Can you work these out from the model? Positions are in its coordinate system, mm. A direction names the side the tool comes from. Give positions to 0.01 mm unless a question says otherwise; leave off trailing zeros. Order: outer loops, then holes, each group sorted by start corner. A loop starts at its lowest first (then second) coordinate and runs counter-clockwise, first axis right, second up. Notation, with made-up numbers: M 13.25,-29.75 L 39.25,-29.75 A23 cw 39.25,3.25 Z; hole C 34.25,-9.5 d6. An arc over 180 degrees is marked long. One line per question, with ' | ' between items. Start each with the question number.
1) Please list where these lines run through material, in increasing order: line 1 along Y through (x, z) = (4, -2); line 2 along Y through (x, z) = (8, 8); line 3 along Y through (x, z) = (3.5, 7.75). Write a range as [from, to].
2) If we section it at C-C, the plane x = 6: State how many separate pieces and enclosed holes the cut face has, plus the area to 3 significant figures.
3) For faces 1 (the flat face through (3.5, 2, -1)), 2 (the flat face through (6, 3.85, -1)), 3 (the flat face through (1.08, 12, 14)), 4 (the flat face through (6, -0.25, -1)), 5 (the flat face through (8.5, 2, -1)), which set-ups out of +Z, -Z, +X, -X, +Y, -Y let a thin tool reach every point of the face, with its end or its side?
4) If we section it at D-D, the plane x = 2.25: Please give me the cut outline in (y, z), plus the area to 3 significant figures.
5) I'm going to push flat-ended pins straight in: pin 1 Ø3 at (y, z) = (1.5, 7) entering from +X; pin 2 Ø0.7 at (y, z) = (8.5, -4.5) entering from +X; pin 3 Ø0.7 at (y, z) = (1.5, -6.5) entering from -X. Where does each tip first touch, or does it pass through?
6) If we section it at B-B, the plane z = 1: Please give me the cut outline in (x, y), plus the area to 3 significant figures.
7) If we section it at A-A, the plane z = -5.4: Please give me the cut outline in (x, y), plus the area to 3 significant figures.
8) Thinking about a two-plate mould opening in Z: for faces 6 (the cylindrical face through (5.9, 15.4, 15.3)), 7 (the flat face through (7, -0.8, 2)), 8 (the cylindrical face through (5.263, 8.596, -4.724)), 9 (the flat face through (6, 17.2, 7)), which applies, +Z half, -Z half, draft (parallel to the pull), parting line (faces both ways), or undercut?
```python
from build123d import *

# Parameters (mm, degrees)
SKETCH001_W      = 9
SKETCH001_H      = 3
EXTRUDE001_DEPTH = 0.8
SKETCH002_W      = 9
SKETCH002_H      = 3
EXTRUDE002_DEPTH = 0.8
EXTRUDE005_DEPTH = 15.15
EXTRUDE004_DEPTH = 21.28
SKETCH003_W      = 15.15
SKETCH003_H      = 21.28
EXTRUDE003_DEPTH = 2.15
EXTRUDE006_DEPTH = 6
EXTRUDE007_DEPTH = 9.84
SKETCH008_W      = 5
SKETCH008_H      = 4.1
EXTRUDE008_DEPTH = 1.8
SKETCH010_R      = 1
EXTRUDE010_DEPTH = 8
SKETCH009_W      = 4.8
SKETCH009_H      = 0.64
EXTRUDE009_DEPTH = 7.2
SKETCH_W         = 12
SKETCH_H         = 17.2
EXTRUDE_DEPTH    = 11


with BuildPart() as extrude001:
    # Sketch001 (on Face1 of Extrude) → Extrude001 (new body)
    with BuildSketch(Plane.XZ):
        with Locations((7.5, 1.5)):
            Rectangle(SKETCH001_W, SKETCH001_H)
    extrude(amount=EXTRUDE001_DEPTH)


with BuildPart() as extrude002:
    # Sketch002 (on Face3 of Extrude) → Extrude002 (new body)
    with BuildSketch(Plane(origin=(0, 17.2, 0), x_dir=(-1, 0, 0), z_dir=(0, 1, 0))):
        with Locations((-7.5, 1.5)):
            Rectangle(SKETCH002_W, SKETCH002_H)
    extrude(amount=EXTRUDE002_DEPTH)


with BuildPart() as extrude005:
    # Sketch005 (on Face3 of Extrude003) → Extrude005 (new body)
    with BuildSketch(Plane.YZ.offset(13.575)):
        Polygon((19.24, 13.15), (17.74, 13.15), (19.24, 12.5), align=None)
        Polygon((-2.04, 13.15), (-0.54, 13.15), (-2.04, 12.5), align=None)
    extrude(amount=-EXTRUDE005_DEPTH)


with BuildPart() as fusion:
    # Sketch004 (on Face4 of Extrude003) → Extrude004 (new body)
    with BuildSketch(Plane(origin=(0, 19.24, 0), x_dir=(-1, 0, 0), z_dir=(0, 1, 0))):
        Polygon((-12.075, 13.15), (-13.575, 12.5), (-13.575, 13.15), align=None)
        Polygon((1.575, 13.15), (1.575, 12.5), (0.075, 13.15), align=None)
    extrude(amount=-EXTRUDE004_DEPTH)

    # Fusion: union Extrude005
    add(extrude005.part)


with BuildPart() as cut:
    # Sketch003 (on Face6 of Extrude) → Extrude003 (new body)
    with BuildSketch(Plane.XY.offset(11)):
        with Locations((6, 8.6)):
            Rectangle(SKETCH003_W, SKETCH003_H)
    extrude(amount=EXTRUDE003_DEPTH)

    # Cut: cut Fusion
    add(fusion.part, mode=Mode.SUBTRACT)


with BuildPart() as extrude006:
    # Sketch006 (on Face2 of Extrude) → Extrude006 (new body)
    with BuildSketch(Plane.YZ.offset(3)):
        Polygon((17.2, 3), (18.2, 7.6), (17.2, 11), (18, 11), (19, 7.6), (18, 3), align=None)
        Polygon((-0.8, 3), (-1.8, 7.6), (-0.8, 11), (0, 11), (-1, 7.6), (0, 3), align=None)
    extrude(amount=EXTRUDE006_DEPTH)


with BuildPart() as extrude007:
    # Sketch007 (on Face4 of Extrude) → Extrude007 (new body)
    with BuildSketch(Plane(origin=(1.08, 0, 0), x_dir=(0, -1, 0), z_dir=(-1, 0, 0))):
        with BuildLine():
            Line((-0.7, 11), (-0.7, 13.3))
            ThreePointArc((-13.9, 17.04), (-7.559803, 14.253048), (-0.7, 13.3))
            ThreePointArc((-13.9, 17.04), (-15.395706, 15.306052), (-16.5, 13.3))
            Line((-16.5, 11), (-16.5, 13.3))
            Line((-16.5, 11), (-0.7, 11))
        make_face()
    extrude(amount=-EXTRUDE007_DEPTH)


with BuildPart() as extrude008:
    # Sketch008 (on Face5 of Extrude) → Extrude008 (new body)
    with BuildSketch(Plane(origin=(0, 0, 0), x_dir=(1, 0, 0), z_dir=(0, 0, -1))):
        with Locations((6, -1.8)):
            Rectangle(SKETCH008_W, SKETCH008_H)
        with Locations((6, -8.6)):
            Rectangle(SKETCH008_W, SKETCH008_H)
        with Locations((6, -15.4)):
            Rectangle(SKETCH008_W, SKETCH008_H)
    extrude(amount=EXTRUDE008_DEPTH)


with BuildPart() as extrude010:
    # Sketch010 (on Face10 of Extrude009) → Extrude010 (new body)
    with BuildSketch(Plane.XZ.offset(-1.48)):
        with Locations((6, -5.4)):
            Circle(SKETCH010_R)
        Polygon((3.6, -9), (4.2, -9), (3.6, -8.4), align=None)
        Polygon((8.4, -9), (7.8, -9), (8.4, -8.4), align=None)
    extrude(amount=-EXTRUDE010_DEPTH)


with BuildPart() as cut001:
    # Sketch009 (on Face6 of Extrude008) → Extrude009 (new body)
    with BuildSketch(Plane(origin=(0, 0, -1.8), x_dir=(1, 0, 0), z_dir=(0, 0, -1))):
        with Locations((6, -1.8)):
            Rectangle(SKETCH009_W, SKETCH009_H)
        with Locations((6, -8.6)):
            Rectangle(SKETCH009_W, SKETCH009_H)
    extrude(amount=EXTRUDE009_DEPTH)

    # Cut001: cut Extrude010
    add(extrude010.part, mode=Mode.SUBTRACT)


with BuildPart() as fusion001:
    # Sketch → Extrude (new body)
    with BuildSketch(Plane.XY):
        with Locations((6, 8.6)):
            Rectangle(SKETCH_W, SKETCH_H)
    extrude(amount=EXTRUDE_DEPTH)

    # Fusion001: union Extrude001, Extrude002, Cut, Extrude006, Extrude007, Extrude008, Cut001
    add(extrude001.part)
    add(extrude002.part)
    add(cut.part)
    add(extrude006.part)
    add(extrude007.part)
    add(extrude008.part)
    add(cut001.part)


solid = fusion001.part
```
Results found:
1) line 1: y = [1.48, 2.12], [8.28, 8.92] | line 2: y = [-1.68, -0.88], [0, 17.2], [18.08, 18.88] | line 3: y = [-1.76, -0.96], [0, 17.2], [18.16, 18.96]
2) separate pieces: 3 | enclosed holes: 2 | area: 304 mm²
3) face 1: -Z, -X, +Y, -Y | face 2: -Z, +X, -X | face 3: +Z, -X, +Y, -Y | face 4: -Z, +X, -X, -Y | face 5: -Z, +X, +Y, -Y
4) outline: M -2.04,11 L 0,11 L 0,0 L 17.2,0 L 17.2,11 L 19.24,11 L 19.24,12.5 L 17.74,13.15 L 16.5,13.15 L 16.5,13.3 A11 ccw 13.9,17.04 A25.16 cw 0.7,13.3 L 0.7,13.15 L -0.54,13.15 L -2.04,12.5 Z | area: 258 mm²
5) pin 1: stops at x = 12 | pin 2: stops at x = 8.4 | pin 3: stops at x = 3.6
6) outline: M 0,0 L 3,0 L 3,-0.8 L 12,-0.8 L 12,18 L 3,18 L 3,17.2 L 0,17.2 Z | area: 221 mm²
7) outline: M 3.6,1.48 L 5,1.48 L 5,2.12 L 3.6,2.12 Z; M 3.6,8.28 L 5,8.28 L 5,8.92 L 3.6,8.92 Z; M 7,1.48 L 8.4,1.48 L 8.4,2.12 L 7,2.12 Z; M 7,8.28 L 8.4,8.28 L 8.4,8.92 L 7,8.92 Z | area: 3.58 mm²
8) face 6: +Z half | face 7: draft | face 8: undercut | face 9: undercut
